Geometry: final body of the model. Coordinates: model frame, mm. Give positions to 0.01 mm unless a question says otherwise; leave off trailing zeros. Write each loop counter-clockwise with the first axis right and the second up, starting at its lowest first coordinate (ties: lowest second). Pieces come first, ordered by that corner, then holes. Notation, with made-up numbers: (77, -38.75) -> (125, -38.75) arc R29 ccw to (125, -0.75) -> close; hole circle Ø7 at (65.5, -36.5). An arc over 180 degrees is marked (long way). Use CSV: the item, a comma, the result in double quotes. Start each with the question number.
1) Material intervals for line 1 (Z direction, x = -13, y = 3.5); line 2 (Z direction, x = -9, y = 3.5); line 3 (Z direction, x = 8.5, y = 6.25), sorted ascending. Write a range as [from, to].
2) Contact query for flat-ended pins moving along their axis: P1, Ø1.5, axis at x = 6, y = 4, coming from the -Z side; P2, Ø3, axis at x = 10, y = 3, coming from the -Z side; P3, Ø5, axis at x = 6.5, z = 5, coming from the -Y side. Output: stop coordinate, or through.
3) Section C-C (z = 15.5). Output: boundary loops of the cut face in (x, y), plus the area to 3 significant figures.
4) Section B-B (x = 0). Output: boundary loops of the cut face in (y, z), plus the area to 3 significant figures.
5) Section A-A (z = 0). Output: boundary loops of the cut face in (x, y).
```python
from build123d import *

# Parameters (mm, degrees)
SKETCH1_R           = 17.78
BOSS_EXTRUDE1_DEPTH = 6.35
CUT_EXTRUDE1_DEPTH  = 7.35


with BuildPart() as part:
    # Sketch1 → Boss-Extrude1 (new body)
    with BuildSketch(Plane(origin=(0, 0, 0), x_dir=(1, 0, 0), z_dir=(0, 1, 0))):
        Circle(SKETCH1_R)
    extrude(amount=BOSS_EXTRUDE1_DEPTH)

    # Sketch2 → Cut-Extrude1 (cut, through all)
    with BuildSketch(Plane(origin=(0, 6.35, 0), x_dir=(1, 0, 0), z_dir=(0, 1, 0))):
        with BuildLine():
            Line((-0.670254455, 13.953911959), (-0.775316452, 12.67631194))
            ThreePointArc((-0.775316452, 12.67631194), (-1.327511483, 12.630428071), (-1.877179521, 12.560501465))
            Line((-1.877179521, 12.560501465), (-2.245573641, 13.788339241))
            ThreePointArc((-2.245573641, 13.788339241), (-2.904526321, 13.664721982), (-3.556789216, 13.509631767))
            Line((-3.556789216, 13.509631767), (-3.393927376, 12.238106756))
            ThreePointArc((-3.393927376, 12.238106756), (-3.924515829, 12.078417757), (-4.447633742, 11.895736803))
            Line((-4.447633742, 11.895736803), (-5.063259395, 13.020149934))
            ThreePointArc((-5.063259395, 13.020149934), (-5.682110904, 12.762230043), (-6.287875221, 12.474915839))
            Line((-6.287875221, 12.474915839), (-5.864207388, 11.265037581))
            ThreePointArc((-5.864207388, 11.265037581), (-6.35, 10.998522628), (-6.823705026, 10.711071362))
            Line((-6.823705026, 10.711071362), (-7.659656416, 11.682917597))
            ThreePointArc((-7.659656416, 11.682917597), (-8.211359975, 11.301967411), (-8.744150906, 10.894986229))
            Line((-8.744150906, 10.894986229), (-8.078193398, 9.799632209))
            ThreePointArc((-8.078193398, 9.799632209), (-8.497958701, 9.437939284), (-8.901547657, 9.058280704))
            Line((-8.901547657, 9.058280704), (-9.921289697, 9.835085701))
            ThreePointArc((-9.921289697, 9.835085701), (-10.381733212, 9.347754571), (-10.818265238, 8.83889344))
            Line((-10.818265238, 8.83889344), (-9.939123592, 7.905935885))
            ThreePointArc((-9.939123592, 7.905935885), (-10.274515829, 7.464872704), (-10.59034994, 7.009599713))
            Line((-10.59034994, 7.009599713), (-11.749315011, 7.557413365))
            ThreePointArc((-11.749315011, 7.557413365), (-12.098374891, 6.985), (-12.419569467, 6.396498594))
            Line((-12.419569467, 6.396498594), (-11.365666392, 5.666712226))
            ThreePointArc((-11.365666392, 5.666712226), (-11.602027312, 5.165555367), (-11.816303113, 4.654565579))
            Line((-11.816303113, 4.654565579), (-13.063838879, 4.949445801))
            ThreePointArc((-13.063838879, 4.949445801), (-13.286259533, 4.316967411), (-13.478078914, 3.674546066))
            Line((-13.478078914, 3.674546066), (-12.295475033, 3.179826051))
            ThreePointArc((-12.295475033, 3.179826051), (-12.422474529, 2.640478473), (-12.52582714, 2.096104594))
            Line((-12.52582714, 2.096104594), (-13.807410301, 2.125163705))
            ThreePointArc((-13.807410301, 2.125163705), (-13.893470878, 1.460262632), (-13.947531638, 0.791998242))
            Line((-13.947531638, 0.791998242), (-12.687912414, 0.55396622))
            ThreePointArc((-12.687912414, 0.55396622), (-12.7, 0), (-12.687912414, -0.55396622))
            Line((-12.687912414, -0.55396622), (-13.947531638, -0.791998242))
            ThreePointArc((-13.947531638, -0.791998242), (-13.893470878, -1.460262632), (-13.807410301, -2.125163705))
            Line((-13.807410301, -2.125163705), (-12.52582714, -2.096104594))
            ThreePointArc((-12.52582714, -2.096104594), (-12.422474529, -2.640478473), (-12.295475033, -3.179826051))
            Line((-12.295475033, -3.179826051), (-13.478078914, -3.674546066))
            ThreePointArc((-13.478078914, -3.674546066), (-13.286259533, -4.316967411), (-13.063838879, -4.949445801))
            Line((-13.063838879, -4.949445801), (-11.816303113, -4.654565579))
            ThreePointArc((-11.816303113, -4.654565579), (-11.602027312, -5.165555367), (-11.365666392, -5.666712226))
            Line((-11.365666392, -5.666712226), (-12.419569467, -6.396498594))
            ThreePointArc((-12.419569467, -6.396498594), (-12.098374891, -6.985), (-11.749315011, -7.557413365))
            Line((-11.749315011, -7.557413365), (-10.59034994, -7.009599713))
            ThreePointArc((-10.59034994, -7.009599713), (-10.274515829, -7.464872704), (-9.939123592, -7.905935885))
            Line((-9.939123592, -7.905935885), (-10.818265238, -8.83889344))
            ThreePointArc((-10.818265238, -8.83889344), (-10.381733212, -9.347754571), (-9.921289697, -9.835085701))
            Line((-9.921289697, -9.835085701), (-8.901547657, -9.058280704))
            ThreePointArc((-8.901547657, -9.058280704), (-8.497958701, -9.437939284), (-8.078193398, -9.799632209))
            Line((-8.078193398, -9.799632209), (-8.744150906, -10.894986229))
            ThreePointArc((-8.744150906, -10.894986229), (-8.211359975, -11.301967411), (-7.659656416, -11.682917597))
            Line((-7.659656416, -11.682917597), (-6.823705026, -10.711071362))
            ThreePointArc((-6.823705026, -10.711071362), (-6.35, -10.998522628), (-5.864207388, -11.265037581))
            Line((-5.864207388, -11.265037581), (-6.287875221, -12.474915839))
            ThreePointArc((-6.287875221, -12.474915839), (-5.682110904, -12.762230043), (-5.063259395, -13.020149934))
            Line((-5.063259395, -13.020149934), (-4.447633742, -11.895736803))
            ThreePointArc((-4.447633742, -11.895736803), (-3.924515829, -12.078417757), (-3.393927376, -12.238106756))
            Line((-3.393927376, -12.238106756), (-3.556789216, -13.509631767))
            ThreePointArc((-3.556789216, -13.509631767), (-2.904526321, -13.664721982), (-2.245573641, -13.788339241))
            Line((-2.245573641, -13.788339241), (-1.877179521, -12.560501465))
            ThreePointArc((-1.877179521, -12.560501465), (-1.327511483, -12.630428071), (-0.775316452, -12.67631194))
            Line((-0.775316452, -12.67631194), (-0.670254455, -13.953911959))
            ThreePointArc((-0.670254455, -13.953911959), (0, -13.97), (0.670254455, -13.953911959))
            Line((0.670254455, -13.953911959), (0.775316452, -12.67631194))
            ThreePointArc((0.775316452, -12.67631194), (1.327511483, -12.630428071), (1.877179521, -12.560501465))
            Line((1.877179521, -12.560501465), (2.245573641, -13.788339241))
            ThreePointArc((2.245573641, -13.788339241), (2.904526321, -13.664721982), (3.556789216, -13.509631767))
            Line((3.556789216, -13.509631767), (3.393927376, -12.238106756))
            ThreePointArc((3.393927376, -12.238106756), (3.924515829, -12.078417757), (4.447633742, -11.895736803))
            Line((4.447633742, -11.895736803), (5.063259395, -13.020149934))
            ThreePointArc((5.063259395, -13.020149934), (5.682110904, -12.762230043), (6.287875221, -12.474915839))
            Line((6.287875221, -12.474915839), (5.864207388, -11.265037581))
            ThreePointArc((5.864207388, -11.265037581), (6.35, -10.998522628), (6.823705026, -10.711071362))
            Line((6.823705026, -10.711071362), (7.659656416, -11.682917597))
            ThreePointArc((7.659656416, -11.682917597), (8.211359975, -11.301967411), (8.744150906, -10.894986229))
            Line((8.744150906, -10.894986229), (8.078193398, -9.799632209))
            ThreePointArc((8.078193398, -9.799632209), (8.497958701, -9.437939284), (8.901547657, -9.058280704))
            Line((8.901547657, -9.058280704), (9.921289697, -9.835085701))
            ThreePointArc((9.921289697, -9.835085701), (10.381733212, -9.347754571), (10.818265238, -8.83889344))
            Line((10.818265238, -8.83889344), (9.939123592, -7.905935885))
            ThreePointArc((9.939123592, -7.905935885), (10.274515829, -7.464872704), (10.59034994, -7.009599713))
            Line((10.59034994, -7.009599713), (11.749315011, -7.557413365))
            ThreePointArc((11.749315011, -7.557413365), (12.098374891, -6.985), (12.419569467, -6.396498594))
            Line((12.419569467, -6.396498594), (11.365666392, -5.666712226))
            ThreePointArc((11.365666392, -5.666712226), (11.602027312, -5.165555367), (11.816303113, -4.654565579))
            Line((11.816303113, -4.654565579), (13.063838879, -4.949445801))
            ThreePointArc((13.063838879, -4.949445801), (13.286259533, -4.316967411), (13.478078914, -3.674546066))
            Line((13.478078914, -3.674546066), (12.295475033, -3.179826051))
            ThreePointArc((12.295475033, -3.179826051), (12.422474529, -2.640478473), (12.52582714, -2.096104594))
            Line((12.52582714, -2.096104594), (13.807410301, -2.125163705))
            ThreePointArc((13.807410301, -2.125163705), (13.893470878, -1.460262632), (13.947531638, -0.791998242))
            Line((13.947531638, -0.791998242), (12.687912414, -0.55396622))
            ThreePointArc((12.687912414, -0.55396622), (12.7, 0), (12.687912414, 0.55396622))
            Line((12.687912414, 0.55396622), (13.947531638, 0.791998242))
            ThreePointArc((13.947531638, 0.791998242), (13.893470878, 1.460262632), (13.807410301, 2.125163705))
            Line((13.807410301, 2.125163705), (12.52582714, 2.096104594))
            ThreePointArc((12.52582714, 2.096104594), (12.422474529, 2.640478473), (12.295475033, 3.179826051))
            Line((12.295475033, 3.179826051), (13.478078914, 3.674546066))
            ThreePointArc((13.478078914, 3.674546066), (13.286259533, 4.316967411), (13.063838879, 4.949445801))
            Line((13.063838879, 4.949445801), (11.816303113, 4.654565579))
            ThreePointArc((11.816303113, 4.654565579), (11.602027312, 5.165555367), (11.365666392, 5.666712226))
            Line((11.365666392, 5.666712226), (12.419569467, 6.396498594))
            ThreePointArc((12.419569467, 6.396498594), (12.098374891, 6.985), (11.749315011, 7.557413365))
            Line((11.749315011, 7.557413365), (10.59034994, 7.009599713))
            ThreePointArc((10.59034994, 7.009599713), (10.274515829, 7.464872704), (9.939123592, 7.905935885))
            Line((9.939123592, 7.905935885), (10.818265238, 8.83889344))
            ThreePointArc((10.818265238, 8.83889344), (10.381733212, 9.347754571), (9.921289697, 9.835085701))
            Line((9.921289697, 9.835085701), (8.901547657, 9.058280704))
            ThreePointArc((8.901547657, 9.058280704), (8.497958701, 9.437939284), (8.078193398, 9.799632209))
            Line((8.078193398, 9.799632209), (8.744150906, 10.894986229))
            ThreePointArc((8.744150906, 10.894986229), (8.211359975, 11.301967411), (7.659656416, 11.682917597))
            Line((7.659656416, 11.682917597), (6.823705026, 10.711071362))
            ThreePointArc((6.823705026, 10.711071362), (6.35, 10.998522628), (5.864207388, 11.265037581))
            Line((5.864207388, 11.265037581), (6.287875221, 12.474915839))
            ThreePointArc((6.287875221, 12.474915839), (5.682110904, 12.762230043), (5.063259395, 13.020149934))
            Line((5.063259395, 13.020149934), (4.447633742, 11.895736803))
            ThreePointArc((4.447633742, 11.895736803), (3.924515829, 12.078417757), (3.393927376, 12.238106756))
            Line((3.393927376, 12.238106756), (3.556789216, 13.509631767))
            ThreePointArc((3.556789216, 13.509631767), (2.904526321, 13.664721982), (2.245573641, 13.788339241))
            Line((2.245573641, 13.788339241), (1.877179521, 12.560501465))
            ThreePointArc((1.877179521, 12.560501465), (1.327511483, 12.630428071), (0.775316452, 12.67631194))
            Line((0.775316452, 12.67631194), (0.670254455, 13.953911959))
            ThreePointArc((0.670254455, 13.953911959), (0, 13.97), (-0.670254455, 13.953911959))
        make_face()
    extrude(amount=-CUT_EXTRUDE1_DEPTH, mode=Mode.SUBTRACT)


solid = part.part
```
Answers follow:
1,line 1,"z = [-12.13, -4.93], [-3.47, -2.11], [-0.61, 0.61], [2.11, 3.47], [4.93, 12.13]"
1,line 2,"z = [-15.33, -9.13], [9.13, 15.33]"
1,line 3,"z = [-15.62, -11.09], [-10.49, -9.44], [9.44, 10.49], [11.09, 15.62]"
2,P1,"stops at z = -16.99"
2,P2,"stops at z = -15.62"
2,P3,"passes through"
3,outline,"(-8.71, 0) -> (8.71, 0) -> (8.71, 6.35) -> (-8.71, 6.35) -> close"
3,area,"111 mm^2"
4,outline,"(0, -17.78) -> (6.35, -17.78) -> (6.35, -13.97) -> (0, -13.97) -> close; (0, 13.97) -> (6.35, 13.97) -> (6.35, 17.78) -> (0, 17.78) -> close"
4,area,"48.4 mm^2"
5,outline,"(-17.78, 0) -> (-12.7, 0) -> (-12.7, 6.35) -> (-17.78, 6.35) -> close; (12.7, 0) -> (17.78, 0) -> (17.78, 6.35) -> (12.7, 6.35) -> close"
